```python
from build123d import *

# Parameters (mm, degrees)
F0_W     = 4.7625
F0_H     = 127
F1_DEPTH = 127
F2_R     = 6.35
F3_DEPTH = 50.8
F4_R     = 3.175


with BuildPart() as f1:
    # F0 (on Top) → F1 (new body)
    with BuildSketch(Plane.XY):
        with Locations((30.95625, -63.5)):
            Rectangle(F0_W, F0_H)
    extrude(amount=F1_DEPTH)

    # F2 (on Right) → F3 (cut, symmetric)
    with BuildSketch(Plane.YZ):
        with Locations((-15.24, 111.76)):
            Circle(F2_R)
        with Locations((-15.24, 60.96)):
            Circle(F2_R)
        Polygon((0, 0), (0, 50.8), (-33.866667, 0), align=None)
        Polygon((-127, 0), (-66.675, 0), (-66.675, 22.225), (-57.15, 22.225), (-38.1, 50.8), (-38.1, 111.125), (-28.934564, 127), (-127, 127), align=None)
    extrude(amount=F3_DEPTH, both=True, mode=Mode.SUBTRACT)

    # F4
    f4_edges = [f1.edges().sort_by_distance(p)[0] for p in [
        (30.95625, -57.15, 22.225),
        (30.95625, -38.1, 50.8),
    ]]
    fillet(f4_edges, radius=F4_R)


solid = f1.part
```
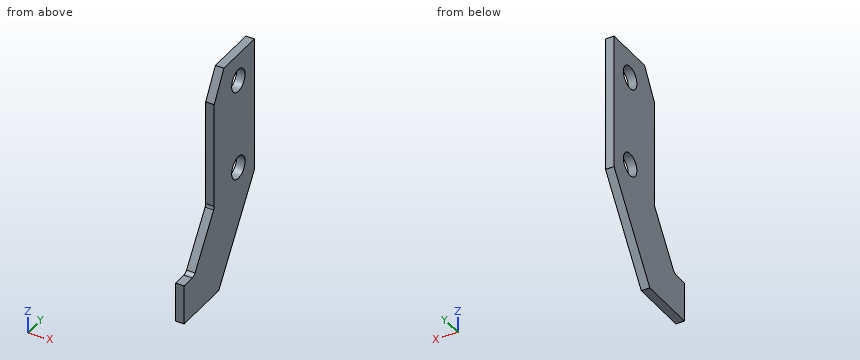
Verification items for the finished model (mm, model axes). Round coordinates to 2 decimals unless told otherwise and drop trailing zeros. Write each loop counter-clockwise with the first axis right and the second up, starting at its lowest first coordinate (ties: lowest second). Pieces come first, ordered by that corner, then holes. Notation, with made-up numbers: (78.25, 46.5) - (126.25, 46.5) arc R19 ccw to (126.25, 63.5) - close; hole circle Ø6 at (-16.5, -14.5). An arc over 180 degrees is marked (long way). Answer as a JSON object with one key per item and string values. Group by question number.
Q1. Section check A-A, the plane x = 31.55. Enter the section's corners in (y, z) (3 decimals).
Q2. Section check B-B, the plane y = -15.24. Enter the section's corners in (x, z) (1 decimal).
Q3. Go/stop test with flat-tipped pins: pin 1 Ø7.5 at (y, z) = (-15.24, 60.96) entering from +X; pin 2 Ø2.5 at (x, y) = (30.5, -64.5) entering from +Z (3 decimals); pin 3 Ø1 at (x, y) = (30, -8.5) entering from -Z; pin 4 Ø1.5 at (x, z) = (32.5, 109.5) entering from -Y. Record where each tip stops, or that it passes through.
Q4. Section check C-C, the plane z = 60.96. Enter the section's corners in (x, y) (1 decimal).
Q5. Thickness scan on line 1 (Z direction, x = 30.25, y = -15.24); line 2 (Z direction, x = 30.55, y = -10.5); line 3 (Y direction, x = 31, z = 60.96). Record the ranges inside material, lowest first.
Found:
{
 "1": {"outline": "(-66.675, 0) - (-33.867, 0) - (0, 50.8) - (0, 127) - (-28.935, 127) - (-38.1, 111.125) - (-38.1, 51.761) arc R3.175 cw to (-38.633, 50) - (-56.207, 23.639) arc R3.175 cw to (-58.849, 22.225) - (-66.675, 22.225) - close; hole circle Ø12.7 at (-15.24, 60.96); hole circle Ø12.7 at (-15.24, 111.76)"},
 "2": {"outline": "(28.6, 27.9) - (33.3, 27.9) - (33.3, 54.6) - (28.6, 54.6) - close; (28.6, 67.3) - (33.3, 67.3) - (33.3, 105.4) - (28.6, 105.4) - close; (28.6, 118.1) - (33.3, 118.1) - (33.3, 127) - (28.6, 127) - close"},
 "3": {"pin 1": "passes through", "pin 2": "stops at z = 22.225", "pin 3": "stops at z = 37.3", "pin 4": "stops at y = -38.1"},
 "4": {"outline": "(28.6, -38.1) - (33.3, -38.1) - (33.3, -21.6) - (28.6, -21.6) - close; (28.6, -8.9) - (33.3, -8.9) - (33.3, 0) - (28.6, 0) - close"},
 "5": {"line 1": "z = 27.94 to 54.61, 67.31 to 105.41, 118.11 to 127", "line 2": "z = 35.05 to 56.73, 65.19 to 107.53, 115.99 to 127", "line 3": "y = -38.1 to -21.59, -8.89 to 0"}
}
